The listing builds one solid part. Answer for the finished solid, in the listing's coordinates (mm). A direction names the side the tool comes from. Give positions to 0.01 mm unless a question says otherwise; leave off trailing zeros. Loops run counter-clockwise (first coordinate to the right, second up) from the corner with the lowest first, then second, coordinate; pieces in that order, holes last. Notation, with made-up numbers: (34, -21.5) -> (61, -21.5) arc R26 cw to (61, -1.5) -> close; hole circle Ø2 at (30.5, 30.5). An arc over 180 degrees is marked (long way). One line per question, with ' | ' between items. Start each with the question number.
from build123d import *

# Parameters (mm, degrees)
SKETCH1_R           = 5
BOSS_EXTRUDE1_DEPTH = 5
BOSS_EXTRUDE2_DEPTH = 40
SKETCH4_W           = 48.223256465
SKETCH4_H           = 80
CUT_EXTRUDE1_DEPTH  = 40
CHAMFER1_SIZE       = 10


with BuildPart() as part:
    # Sketch1 → Boss-Extrude1 (new, symmetric)
    with BuildSketch(Plane.XY):
        with BuildLine():
            Line((-112, 10), (112, 10))
            ThreePointArc((112, 10), (122, 0), (112, -10))
            Line((112, -10), (-112, -10))
            ThreePointArc((-112, -10), (-122, 0), (-112, 10))
        make_face()
        with Locations((-112, 0)):
            Circle(SKETCH1_R, mode=Mode.SUBTRACT)
        with Locations(Location((112, 0, 0), (0, 0, 180))):
            Circle(SKETCH1_R, mode=Mode.SUBTRACT)
    extrude(amount=BOSS_EXTRUDE1_DEPTH, both=True)

    # Sketch2 → Boss-Extrude2 (add)
    with BuildSketch(Plane.XY.offset(5)):
        with BuildLine():
            Line((-112, -10), (112, -10))
            ThreePointArc((112, -10), (122, 0), (112, 10))
            Line((112, 10), (-112, 10))
            ThreePointArc((-112, 10), (-122, 0), (-112, -10))
        make_face()
        with BuildLine():
            Line((-112, -5), (112, -5))
            ThreePointArc((112, -5), (117, 0), (112, 5))
            Line((112, 5), (-112, 5))
            ThreePointArc((-112, 5), (-117, 0), (-112, -5))
        make_face(mode=Mode.SUBTRACT)
    extrude(amount=BOSS_EXTRUDE2_DEPTH)

    # Mirror1: part across plane


with BuildPart() as part_1:
    add(part.part)
    add(part.part.mirror(Plane(origin=(-112, 0, 45), x_dir=(1, 0, 0), z_dir=(0, 0, 1))))

    # Sketch4 → Cut-Extrude1 (cut)
    with BuildSketch(Plane(origin=(0, 10, 0), x_dir=(1, 0, 0), z_dir=(0, 1, 0))):
        with Locations((-116.111628233, -45)):
            Rectangle(SKETCH4_W, SKETCH4_H)
        with Locations((116.111628233, -45)):
            Rectangle(SKETCH4_W, SKETCH4_H)
    extrude(amount=-CUT_EXTRUDE1_DEPTH, mode=Mode.SUBTRACT)

    # Chamfer1
    chamfer1_edges = [part_1.edges().sort_by_distance(p)[0] for p in [
        (-92, 7.5, 5),
        (92, -7.5, 5),
        (92, 7.5, 5),
        (92, -7.5, 85),
        (92, 7.5, 85),
        (-92, -7.5, 85),
        (-92, 7.5, 85),
        (-92, -7.5, 5),
    ]]
    chamfer(chamfer1_edges, length=CHAMFER1_SIZE)

    # Fillet1
    # a fillet whose section is not a circle: 8 mm, written as the material it adds along each edge (its section moved 0.00015 mm through the faces so that the kernel can cut it)
    with BuildSketch(Plane(origin=(-92, -5, 15), x_dir=(4.5266504249621425e-05, 0, 0.9999999989754718), z_dir=(0, -1, 0)), Plane(origin=(-102, -5, 5), x_dir=(0.7071387887142107, 0, 0.7070747722099827), z_dir=(0, -1, 0)), Plane(origin=(-92, -5, 75), x_dir=(-0.707074772209981, 0, 0.7071387887142122), z_dir=(0, -1, 0)), Plane(origin=(-92, 10, 75), x_dir=(-0.707074772209981, 0, 0.7071387887142122), z_dir=(0, -1, 0)), Plane(origin=(102, 10, 85), x_dir=(-0.7071387887142122, 0, -0.707074772209981), z_dir=(0, -1, 0)), Plane(origin=(-102, 10, 5), x_dir=(0.7071387887142107, 0, 0.7070747722099827), z_dir=(0, -1, 0)), Plane(origin=(-92, 10, 15), x_dir=(4.5266504249621425e-05, 0, 0.9999999989754718), z_dir=(0, -1, 0))) as fillet1_piece_1:
        with BuildLine():
            add(Edge.make_bspline([(3.313708502, 0), (2.707126731, -2.7458e-05), (2.10054496, -5.4916e-05), (0.747296328, 0.113741147), (-0.448046284, 0.608804877), (-1.485482876, 1.485136275), (-1.914420376, 1.914034943), (-2.343357875, 2.342933611)], knots=[0, 0, 0, 0, 0, 0, 0.5, 0.5, 1, 1, 1, 1, 1, 1], degree=5))
            Line((-2.343357875, 2.342933611), (-2.456489839, 2.229791405))
            ThreePointArc((-2.456489839, 2.229791405), (-1.284757871, 1.058377635), (-0.113131964, -0.113142206))
            Line((-0.113131964, -0.113142206), (7.243e-06, -0.16))
            ThreePointArc((7.243e-06, -0.16), (1.65686149, -0.159925), (3.313715745, -0.16))
            Line((3.313715745, -0.16), (3.313708502, 0))
        make_face()
    extrude(amount=5)
    with BuildSketch(Plane(origin=(92, -5, 15), x_dir=(-4.526650424962133e-05, 0, 0.9999999989754718), z_dir=(0, -1, 0)), Plane(origin=(92, -5, 75), x_dir=(0.707074772209981, 0, 0.7071387887142122), z_dir=(0, -1, 0)), Plane(origin=(102, -5, 85), x_dir=(0.9999999989754718, 0, 4.526650424962133e-05), z_dir=(0, -1, 0)), Plane(origin=(-102, -5, 85), x_dir=(0.7071387887142122, 0, -0.707074772209981), z_dir=(0, -1, 0)), Plane(origin=(102, -5, 5), x_dir=(-0.7071387887142124, 0, 0.7070747722099809), z_dir=(0, -1, 0)), Plane(origin=(-102, 10, 85), x_dir=(0.7071387887142122, 0, -0.707074772209981), z_dir=(0, -1, 0)), Plane(origin=(92, 10, 75), x_dir=(0.707074772209981, 0, 0.7071387887142122), z_dir=(0, -1, 0)), Plane(origin=(92, 10, 15), x_dir=(-4.526650424962133e-05, 0, 0.9999999989754718), z_dir=(0, -1, 0)), Plane(origin=(102, 10, 5), x_dir=(-0.7071387887142124, 0, 0.7070747722099809), z_dir=(0, -1, 0))) as fillet1_piece_2:
        with BuildLine():
            add(Edge.make_bspline([(3.313708502, 0), (2.707126731, 2.7458e-05), (2.10054496, 5.4916e-05), (0.747296328, -0.113741147), (-0.448046284, -0.608804877), (-1.485482876, -1.485136275), (-1.914420376, -1.914034943), (-2.343357875, -2.342933611)], knots=[0, 0, 0, 0, 0, 0, 0.5, 0.5, 1, 1, 1, 1, 1, 1], degree=5))
            Line((-2.343357875, -2.342933611), (-2.456489839, -2.229791405))
            ThreePointArc((-2.456489839, -2.229791405), (-1.284757871, -1.058377635), (-0.113131964, 0.113142206))
            Line((-0.113131964, 0.113142206), (7.243e-06, 0.16))
            ThreePointArc((7.243e-06, 0.16), (1.65686149, 0.159925), (3.313715745, 0.16))
            Line((3.313715745, 0.16), (3.313708502, 0))
        make_face()
    extrude(amount=5)


solid = part_1.part
1. The part is cut by section C-C (x = 65). Write down the section's boundary in (y, z).
2. The part is cut by section A-A (z = 62.5). Write down the section's boundary in (x, y), plus the area to 3 significant figures.
3. Each of these flat-tipped pins is pushed along its axis until it touches: pin 1 Ø4 at (y, z) = (-7, 67.5) entering from +X; pin 2 Ø9 at (x, y) = (112, 0) entering from -Z (3 decimals); pin 3 Ø4 at (y, z) = (-7, 33) entering from -X. Where does it stop, or does it pass through?
4. Straight lines are drawn through the part: L1, parallel to Z at x = 55, y = 0.75; L2, parallel to Y at x = 43, z = 27.5; L3, parallel to X at y = -8, z = 70.5. For each, find the intervals that lie inside material, in ascending order.
5. Determine the mould class of faces 4 (the flat face through (2, 0, -5)), 5 (the flat face through (-1, -5, 46)), 6 (the flat face through (2, 10, 46)) for opening direction Y: released by +Y, released by -Y, zero draft, split by the parting line, or undercut.
6. For faces 1 (the flat face through (97, 8, 10)), 2 (the flat face through (-97, -7, 10)), 3 (the flat face through (-6, 5, 40)), determine the directions among +Z, -Z, +X, -X, +Y, -Y from which every point of the face is accessible in a straight line to the end or side of a thin tool.
7. The part is cut by section B-B (y = 0). Write down the section's boundary in (x, z).
8. The part is cut by section D-D (z = 2). Write down the section's boundary in (x, y), plus the area to 3 significant figures.
Check sheet entries:
1) outline: (-10, -5) -> (10, -5) -> (10, 95) -> (-10, 95) -> close; hole (-5, 5) -> (5, 5) -> (5, 85) -> (-5, 85) -> close
2) outline: (-92, -10) -> (92, -10) -> (92, -5) -> (-92, -5) -> close; (-92, 5) -> (92, 5) -> (92, 10) -> (-92, 10) -> close | area: 1,840 mm^2
3) pin 1: stops at x = 92 | pin 2: passes through | pin 3: stops at x = -92
4) L1: z = -5 to 5, 85 to 95 | L2: y = -10 to -5, 5 to 10 | L3: x = -92 to 92
5) face 4: zero draft | face 5: undercut | face 6: released by +Y
6) face 1: +X, +Y, -Y | face 2: -X, +Y, -Y | face 3: +X, -X
7) outline: (-122, -5) -> (-117, -5) -> (-117, 5) -> (-122, 5) -> close; (-122, 85) -> (-117, 85) -> (-117, 95) -> (-122, 95) -> close; (-107, -5) -> (107, -5) -> (107, 5) -> (-107, 5) -> close; (-107, 85) -> (107, 85) -> (107, 95) -> (-107, 95) -> close; (117, -5) -> (122, -5) -> (122, 5) -> (117, 5) -> close; (117, 85) -> (122, 85) -> (122, 95) -> (117, 95) -> close
8) outline: (-112, -10) -> (112, -10) arc R10 ccw to (112, 10) -> (-112, 10) arc R10 ccw to start; hole circle Ø10 at (-112, 0); hole circle Ø10 at (112, 0) | area: 4,640 mm^2
